Check sheet for the modelled part. Datum: model origin and axes. Units: mm. Face numbers are marked on the shaded views. A direction names the side the tool comes from. Round coordinates to 2 decimals unless told otherwise and drop trailing zeros. Order: outer loops, then holes, each group sorted by start corner. A loop starts at its lowest first (then second) coordinate and runs counter-clockwise, first axis right, second up. Notation, with made-up numbers: (76.5, 55) -> (90.5, 55) arc R19 ccw to (90.5, 67) -> close; hole circle Ø2 at (-21.5, -16). An arc over 180 degrees is marked (long way). Answer as CSV lines item,"result". Start each with the question number.
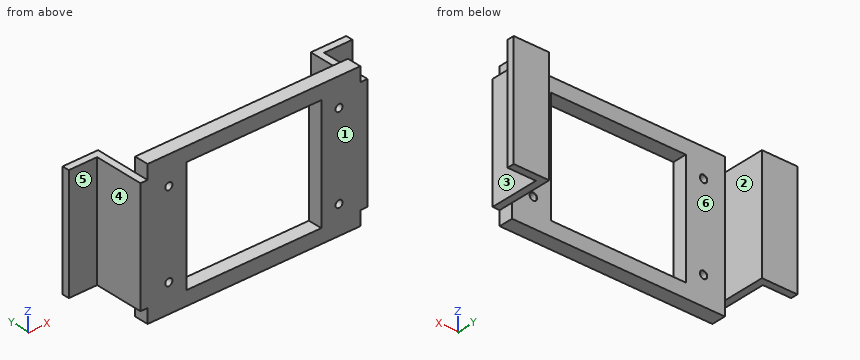
from build123d import *

# Parameters (mm, degrees)
SKETCH_1_W                      = 32
SKETCH_1_H                      = 16
EXTRUDE_1_DEPTH                 = 2
SKETCH_2_W                      = 1
SKETCH_2_H                      = 16
EXTRUDE_2_DEPTH                 = 6
SKETCH_3_W                      = 1
SKETCH_3_H                      = 16
EXTRUDE_3_DEPTH                 = 6
SKETCH_4_W                      = 16
SKETCH_4_H                      = 1
EXTRUDE_4_DEPTH                 = 4
SKETCH_5_W                      = 16
SKETCH_5_H                      = 1
EXTRUDE_5_DEPTH                 = 4
HOLE_WIZARD_1_0_1_1_D           = 1
HOLE_WIZARD_1_0_1_1_CSINK_D     = 1.05
HOLE_WIZARD_1_0_1_1_CSINK_ANGLE = 90
SKETCH_14_W                     = 29.99841147
SKETCH_14_H                     = 2
EXTRUDE_6_DEPTH                 = 2
SKETCH_15_W                     = 29.99841147
SKETCH_15_H                     = 2
EXTRUDE_7_DEPTH                 = 2
SKETCH_16_W                     = 19
SKETCH_16_H                     = 16
CUT_EXTRUDE_1_DEPTH             = 2


with BuildPart() as part:
    # 草图1 → 凸台-拉伸1 (new body)
    with BuildSketch(Plane(origin=(0, 0, 0), x_dir=(1, 0, 0), z_dir=(0, 1, 0))):
        Rectangle(SKETCH_1_W, SKETCH_1_H)
    extrude(amount=EXTRUDE_1_DEPTH)

    # 草图2 → 凸台-拉伸2 (add)
    with BuildSketch(Plane(origin=(0, 2, 0), x_dir=(1, 0, 0), z_dir=(0, 1, 0))):
        with Locations((-15.5, 0)):
            Rectangle(SKETCH_2_W, SKETCH_2_H)
    extrude(amount=EXTRUDE_2_DEPTH)

    # 草图3 → 凸台-拉伸3 (add)
    with BuildSketch(Plane(origin=(0, 2, 0), x_dir=(1, 0, 0), z_dir=(0, 1, 0))):
        with Locations((15.5, 0)):
            Rectangle(SKETCH_3_W, SKETCH_3_H)
    extrude(amount=EXTRUDE_3_DEPTH)

    # 草图4 → 凸台-拉伸4 (add)
    with BuildSketch(Plane.ZY.offset(16)):
        with Locations((0, 7.5)):
            Rectangle(SKETCH_4_W, SKETCH_4_H)
    extrude(amount=EXTRUDE_4_DEPTH)

    # 草图5 → 凸台-拉伸5 (add)
    with BuildSketch(Plane(origin=(16, 0, 0), x_dir=(0, 0, -1), z_dir=(1, 0, 0))):
        with Locations((0, 7.5)):
            Rectangle(SKETCH_5_W, SKETCH_5_H)
    extrude(amount=EXTRUDE_5_DEPTH)

    # Ø1.0 (1) 直径孔1 (through all)
    with Locations(Plane(origin=(0, 2, 0), x_dir=(1, 0, 0), z_dir=(0, 1, 0))):
        with Locations((-12, 6), (-12, -6), (12, -6), (12, 6)):
            CounterSinkHole(HOLE_WIZARD_1_0_1_1_D / 2, HOLE_WIZARD_1_0_1_1_CSINK_D / 2, counter_sink_angle=HOLE_WIZARD_1_0_1_1_CSINK_ANGLE)

    # 草图14 → 凸台-拉伸6 (add)
    with BuildSketch(Plane(origin=(0, 0, -8), x_dir=(-1, 0, 0), z_dir=(0, 0, -1))):
        with Locations((-0.000794265, 1)):
            Rectangle(SKETCH_14_W, SKETCH_14_H)
    extrude(amount=EXTRUDE_6_DEPTH)

    # 草图15 → 凸台-拉伸7 (add)
    with BuildSketch(Plane.XY.offset(8)):
        with Locations((-0.000794265, 1)):
            Rectangle(SKETCH_15_W, SKETCH_15_H)
    extrude(amount=EXTRUDE_7_DEPTH)

    # 草图16 → 切除-拉伸1 (cut)
    with BuildSketch(Plane(origin=(0, 2, 0), x_dir=(1, 0, 0), z_dir=(0, 1, 0))):
        Rectangle(SKETCH_16_W, SKETCH_16_H)
    extrude(amount=-CUT_EXTRUDE_1_DEPTH, mode=Mode.SUBTRACT)


solid = part.part
1) Section check B-B on z = 6. Record the cut outline in (x, y) (3 decimals), then the cut area to 3 significant figures.
2) Depth check by flat-ended pin: pin 1 Ø3.5 at (y, z) = (2, -3) entering from -X; pin 2 Ø3 at (y, z) = (5, 2) entering from +X; pin 3 Ø2 at (y, z) = (1, -9.5) entering from +X; pin 4 Ø10 at (x, z) = (2.5, -2) entering from -Y. Enter the tip coordinate at first touch or a pass-through.
3) Section check A-A on x = -7.5. Record the cut outline in (y, z).
4) Material ranges on line 1 along Z through (x, y) = (-12, 1.65); line 2 along X through (y, z) = (1, -6); line 3 along Z through (x, y) = (3, 0.5), recorded low to high.
5) Section check D-D on x = 12. Record the cut outline in (y, z) (3 decimals).
6) Access from +Z, -Z, +X, -X, +Y, -Y to the whole of each face (thin tool, end or side, straight path). Record for the marked faces 1 and 2.
7) Mould release check, pull along X, two halves, no side actions. Record for the marked faces 3, 4, 5 and 6: released by +X, released by -X, zero draft, split by the parting line, or undercut.
8) Section check C-C on y = 3.75. Record the cut outline in (x, z), then the cut area to 3 significant figures.
Solutions:
1,outline,"(-20, 7) -> (-16, 7) -> (-16, 0) -> (-12.5, 0) -> (-12.5, 1.975) -> (-12.525, 2) -> (-15, 2) -> (-15, 8) -> (-20, 8) -> close; (-11.5, 0) -> (-9.5, 0) -> (-9.5, 2) -> (-11.475, 2) -> (-11.5, 1.975) -> close; (9.5, 0) -> (11.5, 0) -> (11.5, 1.975) -> (11.475, 2) -> (9.5, 2) -> close; (12.5, 0) -> (16, 0) -> (16, 7) -> (20, 7) -> (20, 8) -> (15, 8) -> (15, 2) -> (12.525, 2) -> (12.5, 1.975) -> close"
1,area,"42.0 mm^2"
2,pin 1,"stops at x = -16"
2,pin 2,"stops at x = 16"
2,pin 3,"stops at x = 15"
2,pin 4,"passes through"
3,outline,"(0, -10) -> (2, -10) -> (2, -8) -> (0, -8) -> close; (0, 8) -> (2, 8) -> (2, 10) -> (0, 10) -> close"
4,line 1,"z = -10 to -6.5, -5.5 to 5.5, 6.5 to 10"
4,line 2,"x = -16 to -12.5, -11.5 to -9.5, 9.5 to 11.5, 12.5 to 16"
4,line 3,"z = -10 to -8, 8 to 10"
5,outline,"(0, -10) -> (2, -10) -> (2, -6.525) -> (1.975, -6.5) -> (0, -6.5) -> close; (0, -5.5) -> (1.975, -5.5) -> (2, -5.475) -> (2, 5.475) -> (1.975, 5.5) -> (0, 5.5) -> close; (0, 6.5) -> (1.975, 6.5) -> (2, 6.525) -> (2, 10) -> (0, 10) -> close"
6,face 1,"+Z, -Z, +X, -X, -Y"
6,face 2,"+Z, -Z, +Y"
7,face 3,"released by +X"
7,face 4,"released by -X"
7,face 5,"zero draft"
7,face 6,"undercut"
8,outline,"(-16, -8) -> (-15, -8) -> (-15, 8) -> (-16, 8) -> close; (15, -8) -> (16, -8) -> (16, 8) -> (15, 8) -> close"
8,area,"32.0 mm^2"
